Here's how the part is built. I have some questions about the finished solid (model axes, mm). Give positions to 0.01 mm unless a question says otherwise; leave off trailing zeros. Write each loop counter-clockwise with the first axis right and the second up, starting at its lowest first coordinate (ties: lowest second). Pieces come first, ordered by that corner, then holes. Notation, with made-up numbers: (-15.75, 85.25) - (23.25, 85.25) arc R27 cw to (23.25, 107.25) - close; hole circle Ø5 at (82.5, -19.5). An arc over 180 degrees is marked (long way). Write each question's results on one line, items separated by ' | '. Start each with the question number.
Item 1: Suppose I cut it at C-C on x = 1. List the corners of the cut face in (y, z) for me, then the cut area to 3 significant figures.
Item 2: Suppose I cut it at D-D on y = 0.5. Count the separate pieces of the cut face and the enclosed holes in it, then the cut area to 3 significant figures.
Item 3: Suppose I cut it at A-A on z = 24.5. List the corners of the cut face in (x, y) for me, then the cut area to 3 significant figures.
Item 4: Suppose I cut it at B-B on z = 12.5. List the corners of the cut face in (x, y) for me, then the cut area to 3 significant figures.
Item 5: Please list where these lines run through material, in increasing order: line 1 along Z through (x, y) = (-32, 0.1); line 2 along X through (y, z) = (1.4, 25); line 3 along X through (y, z) = (1.3, 13).
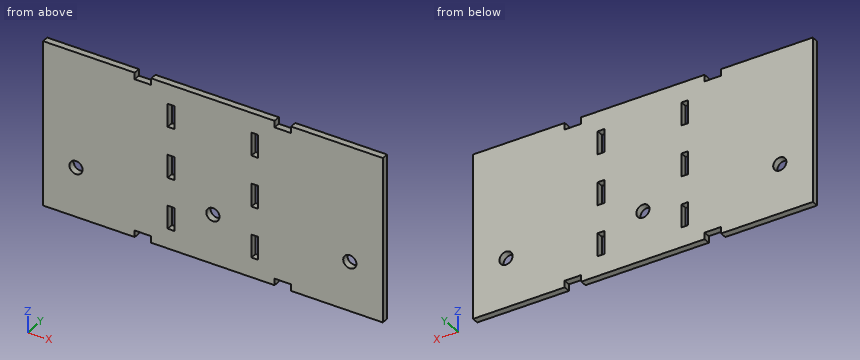
```python
from build123d import *

# Parameters (mm, degrees)
SKETCH1_W           = 2
SKETCH1_H           = 7
SKETCH1_R           = 2
BOSS_EXTRUDE1_DEPTH = 2


with BuildPart() as part:
    # Sketch1 → Boss-Extrude1 (new body)
    with BuildSketch(Plane(origin=(0, 0, 0), x_dir=(1, 0, 0), z_dir=(0, 1, 0))):
        Polygon((-42.999453113, 2.019339096), (-70.799453113, 2.019339096), (-70.799453113, -47.980660904), (-42.999453113, -47.980660904), (-42.999453113, -45.980660904), (-37.999453113, -45.980660904), (-37.999453113, -47.980660904), (-0.599453113, -47.980660904), (-0.599453113, -45.980660904), (4.400546887, -45.980660904), (4.400546887, -47.980660904), (32.200546887, -47.980660904), (32.200546887, 2.019339096), (4.400546887, 2.019339096), (4.400546887, 0.019339096), (-0.599453113, 0.019339096), (-0.599453113, 2.019339096), (-37.999453113, 2.019339096), (-37.999453113, 0.019339096), (-42.999453113, 0.019339096), align=None)
        with Locations((-31.999453113, -38.480660904)):
            Rectangle(SKETCH1_W, SKETCH1_H, mode=Mode.SUBTRACT)
        with Locations((-6.599453113, -38.480660904)):
            Rectangle(SKETCH1_W, SKETCH1_H, mode=Mode.SUBTRACT)
        with Locations(Location((-60.799453113, -12.980660904, 0), (0, 0, 270))):
            Circle(SKETCH1_R, mode=Mode.SUBTRACT)
        with Locations((-31.999453113, -22.980660904)):
            Rectangle(SKETCH1_W, SKETCH1_H, mode=Mode.SUBTRACT)
        with Locations(Location((-19.299453113, -12.980660904, 0), (0, 0, 270))):
            Circle(SKETCH1_R, mode=Mode.SUBTRACT)
        with Locations((-31.999453113, -7.480660904)):
            Rectangle(SKETCH1_W, SKETCH1_H, mode=Mode.SUBTRACT)
        with Locations((-6.599453113, -22.980660904)):
            Rectangle(SKETCH1_W, SKETCH1_H, mode=Mode.SUBTRACT)
        with Locations(Location((22.200546887, -12.980660904, 0), (0, 0, 270))):
            Circle(SKETCH1_R, mode=Mode.SUBTRACT)
        with Locations((-6.599453113, -7.480660904)):
            Rectangle(SKETCH1_W, SKETCH1_H, mode=Mode.SUBTRACT)
    extrude(amount=BOSS_EXTRUDE1_DEPTH)


solid = part.part
```
Checked values:
1) outline: (0, -0.02) - (2, -0.02) - (2, 45.98) - (0, 45.98) - close | area: 92.0 mm^2
2) separate pieces: 1 | enclosed holes: 9 | area: 4,990 mm^2
3) outline: (-70.8, 0) - (-33, 0) - (-33, 2) - (-70.8, 2) - close; (-31, 0) - (-7.6, 0) - (-7.6, 2) - (-31, 2) - close; (-5.6, 0) - (32.2, 0) - (32.2, 2) - (-5.6, 2) - close | area: 198 mm^2
4) outline: (-70.8, 0) - (-62.74, 0) - (-62.74, 2) - (-70.8, 2) - close; (-58.86, 0) - (-21.24, 0) - (-21.24, 2) - (-58.86, 2) - close; (-17.36, 0) - (20.26, 0) - (20.26, 2) - (-17.36, 2) - close; (24.14, 0) - (32.2, 0) - (32.2, 2) - (24.14, 2) - close | area: 183 mm^2
5) line 1: z = -2.02 to 3.98, 10.98 to 19.48, 26.48 to 34.98, 41.98 to 47.98 | line 2: x = -70.8 to -33, -31 to -7.6, -5.6 to 32.2 | line 3: x = -70.8 to -62.8, -58.8 to -21.3, -17.3 to 20.2, 24.2 to 32.2
